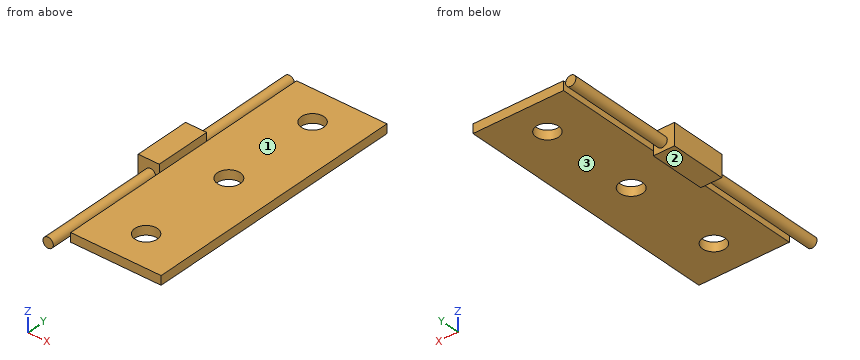
```python
from build123d import *

# Parameters (mm, degrees)
CROQUIS1_W                   = 30
CROQUIS1_H                   = 89
SALIENTE_EXTRUIR1_DEPTH      = 3
CROQUIS2_R                   = 3.800850318
CROQUIS2_R_2                 = 3.742975761
CORTAR_EXTRUIR1_DEPTH        = 3
CROQUIS3_W                   = 7.223510215
CROQUIS3_H                   = 18.667669577
SALIENTE_EXTRUIR2_DEPTH      = 7
SALIENTE_EXTRUIR3_DEPTH      = 36
SALIENTE_EXTRUIR3_DEPTH_BACK = 59
CROQUIS4_R                   = 1.707521399


with BuildPart() as part:
    # Croquis1 → Saliente-Extruir1 (new body)
    with BuildSketch(Plane.XY):
        Rectangle(CROQUIS1_W, CROQUIS1_H)
    extrude(amount=SALIENTE_EXTRUIR1_DEPTH)

    # Croquis2 → Cortar-Extruir1 (cut)
    with BuildSketch(Plane.XY.offset(3)):
        Circle(CROQUIS2_R)
        with Locations((0, 32.997286313)):
            Circle(CROQUIS2_R_2)
        with Locations((0, -32.603288865)):
            Circle(CROQUIS2_R_2)
    extrude(amount=-CORTAR_EXTRUIR1_DEPTH, mode=Mode.SUBTRACT)

    # Croquis3 → Saliente-Extruir2 (add)
    with BuildSketch(Plane.ZY.offset(15)):
        with Locations((2.087224579, -0.259009368)):
            Rectangle(CROQUIS3_W, CROQUIS3_H)
    extrude(amount=SALIENTE_EXTRUIR2_DEPTH)

    # Croquis4 → Saliente-Extruir3 (add, two sides: drawn at the far end of the back side and taken through both)
    with BuildSketch(Plane(origin=(0, 9.074825421, 0), x_dir=(1, 0, 0), z_dir=(0, 1, 0)).offset(-SALIENTE_EXTRUIR3_DEPTH_BACK)):
        with Locations(Location((-17.910478142, -1.422079338, 0), (0, 0, 180))):
            Circle(CROQUIS4_R)
    extrude(amount=SALIENTE_EXTRUIR3_DEPTH + SALIENTE_EXTRUIR3_DEPTH_BACK)


solid = part.part
```
Verification items for the finished model (mm, model axes). Face numbers are marked on the shaded views. A direction names the side the tool comes from. Coordinates: 2 decimals unless noted, no trailing zeros. Write each loop counter-clockwise with the first axis right and the second up, starting at its lowest first coordinate (ties: lowest second). Pieces come first, ordered by that corner, then holes. Notation, with made-up numbers: M 9.25,77.25 L 68.25,77.25 A18 ccw 68.25,103.25 Z; hole C -35.75,16.25 d5. An arc over 180 degrees is marked long. Answer as a JSON object with one key per item and string values. Group by question number.
(1) Cross-section at A-A, the plane y = 0. Record the cut outline in (x, z), and give its area (3 significant figures).
(2) Cross-section at C-C, the plane y = -33.5. Record the cut outline in (x, z).
(3) Cross-section at B-B, the plane x = 0. Record the cut outline in (y, z).
(4) Cross-section at D-D, the plane x = 11.5. Record the cut outline in (y, z), and give its area (3 significant figures).
(5) Material ranges on line 1 (Y direction, x = 0, z = 0.7); line 2 (Y direction, x = -3, z = 2); line 3 (Y direction, x = -17.5, z = 4), recorded low to high.
(6) Tool access check on the marked faces 1, 2 and 3. Record the directions out of +Z, -Z, +X, -X, +Y, -Y that give a thin tool (end or side, any length) a straight path to the whole face; none if there is none.
(7) Gauge pin test, flat ends, axial feed: pin 1 (2.5 mm diameter, centred on x = 2, z = 1, fed in from +Y); pin 2 (1.5 mm diameter, centred on y = -29.5, z = 1, fed in from -X); pin 3 (8 mm diameter, centred on x = 11, y = 32.5, fed in from +Z). Record the tip position at first contact, or that the pin passes through.
Reply:
{
 "1": {"outline": "M -22,-1.52 L -15,-1.52 L -15,0 L -3.8,0 L -3.8,3 L -15,3 L -15,5.7 L -22,5.7 Z; M 3.8,0 L 15,0 L 15,3 L 3.8,3 Z", "area": "118 mm²"},
 "2": {"outline": "C -17.91,1.42 d3.42; M -15,0 L -3.63,0 L -3.63,3 L -15,3 Z; M 3.63,0 L 15,0 L 15,3 L 3.63,3 Z"},
 "3": {"outline": "M -44.5,0 L -36.35,0 L -36.35,3 L -44.5,3 Z; M -28.86,0 L -3.8,0 L -3.8,3 L -28.86,3 Z; M 3.8,0 L 29.25,0 L 29.25,3 L 3.8,3 Z; M 36.74,0 L 44.5,0 L 44.5,3 L 36.74,3 Z"},
 "4": {"outline": "M -44.5,0 L 44.5,0 L 44.5,3 L -44.5,3 Z", "area": "267 mm²"},
 "5": {"line 1": "-44.5 to -36.35, -28.86 to -3.8, 3.8 to 29.25, 36.74 to 44.5", "line 2": "-44.5 to -34.84, -30.37 to -2.33, 2.33 to 30.76, 35.24 to 44.5", "line 3": "-9.59 to 9.07"},
 "6": {"face 1": "+Z, +X, +Y, -Y", "face 2": "-Z, +X, -X, +Y, -Y", "face 3": "-Z, +X, +Y, -Y"},
 "7": {"pin 1": "y = 44.5", "pin 2": "x = -19.62", "pin 3": "z = 3"}
}
